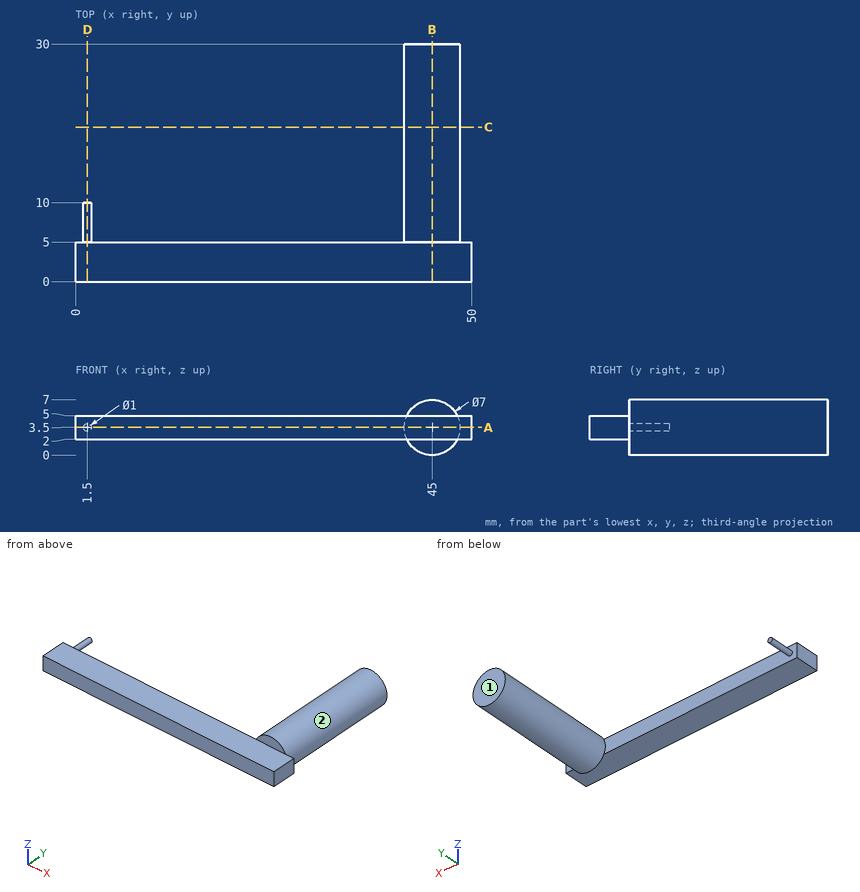
Geometry: see drawing. Coordinates: mm, zero at the bounding-box minimum. A direction names the side the tool comes from. Round coordinates to 2 decimals unless told otherwise and drop trailing zeros. Order: outer loops, then holes, each group sorted by start corner. A loop starts at its lowest first (then second) coordinate and runs counter-clockwise, first axis right, second up. Notation, with made-up numbers: (6, 57) -> (26, 57) arc R11 ccw to (26, 75) -> close; hole circle Ø9 at (80.25, -11). An arc over 180 degrees is marked (long way). Use CSV: the item, a comma, the result in double quotes.
(1) Access query for the marked faces 1 and 2. Directions: +Z, -Z, +X, -X, +Y, -Y. A direction counts if a zero-diameter tool reaches every point of the face in a straight line with its end or side. Return the directions, or none.
Report:
face 1,"+Z, -Z, +X, -X, +Y"
face 2,"+Y"
(2) Ray query, L1, parallel to X at y = 13, z = 2; L2, parallel to Y at x = 9, z = 3.75; L3, parallel to Z at x = 7.5, y = 4. Return the intervals inside material, ascending.
Report:
L1,"41.84 to 48.16"
L2,"0 to 5"
L3,"2 to 5"
(3) Section C-C on y = 19.5. Return the cut outline in (x, z).
Report:
outline,"circle Ø7 at (45, 3.5)"
(4) Section A-A on z = 3.5. Return the cut outline in (x, y).
Report:
outline,"(0, 0) -> (50, 0) -> (50, 5) -> (48.5, 5) -> (48.5, 30) -> (41.5, 30) -> (41.5, 5) -> (2, 5) -> (2, 10) -> (1, 10) -> (1, 5) -> (0, 5) -> close"
(5) Section B-B on x = 45. Return the cut outline in (y, z).
Report:
outline,"(0, 2) -> (5, 2) -> (5, 0) -> (30, 0) -> (30, 7) -> (5, 7) -> (5, 5) -> (0, 5) -> close"
(6) Section D-D on x = 1.5. Return the cut outline in (y, z), and give its area (3 significant figures).
Report:
outline,"(0, 2) -> (5, 2) -> (5, 3) -> (10, 3) -> (10, 4) -> (5, 4) -> (5, 5) -> (0, 5) -> close"
area,"20.0 mm^2"
(7) First-contact query: pin 1 Ø0.9 at (x, z) = (49, 3) entering from +Y; pin 2 Ø5.5 at (x, y) = (35.5, 2) entering from -Z; pin 3 Ø2 at (y, z) = (15.5, 1.5) entering from +X. Flat tips, straight axial feed; report the tip coordinate or a pass-through.
Report:
pin 1,"y = 5"
pin 2,"z = 2"
pin 3,"x = 48.35"
